Geometry check sheet. Reference: the model listing, model coordinates, mm. A direction names the side the tool comes from. Give positions to 0.01 mm unless a question says otherwise; leave off trailing zeros. Write each loop counter-clockwise with the first axis right and the second up, starting at its lowest first coordinate (ties: lowest second). Pieces come first, ordered by that corner, then holes. Notation, with made-up numbers: (20, -2.75) -> (67, -2.75) arc R28 ccw to (67, 32.25) -> close; hole circle Ø11 at (-39, 83.25). An arc over 180 degrees is marked (long way). Write item = value, one per line. Start each with the question number.
1. Thickness scan on line 1 along X through (y, z) = (89, -13.75); line 2 along X through (y, z) = (20.5, -13). Record the ranges inside material, lowest first.
2. Set-up check for faces 1 (the flat face through (-13, 62, -25)), 2 (the flat face through (-12, 65, -22)): record each of +Z, -Z, +X, -X, +Y, -Y from which the full face is reachable in a straight line by a thin tool's end or side.
3. Depth check by flat-ended pin: P1, Ø1.5, axis at x = -17, z = -2.5, coming from the -Y side. Enter the tip coordinate at first touch or a pass-through.
4. Mould release check, pull along X, two halves, no side actions. Record for faces 3 (the flat face through (-25, 74, -12)), 4 (the flat face through (0, 87, -13)), 5 (the flat face through (-22, 74, -13)): pulls with the +X half, pulls with the -X half, needs draft (parallel to the pull), parting line crosses it, or undercut.
5. Cross-section at B-B, the plane z = -7.25. Record the cut outline in (x, y).
6. Cross-section at A-A, the plane x = -9.75. Record the cut outline in (y, z), plus the area to 4 significant figures.
7. Cross-section at C-C, the plane y = 26.5. Record the cut outline in (x, z).
Autodesk Inventor part; units mm, degrees
ref_plane "YZ Plane" through (0, 0, 0) normal (1, 0, 0) x (0, 1, 0)
ref_plane "XZ Plane" through (0, 0, 0) normal (0, 1, 0) x (-1, 0, 0)
ref_plane "XY Plane" through (0, 0, 0) normal (0, 0, 1) x (1, 0, 0)
sketch "Sketch1" plane through (0, 0, 0) normal (0, 1, 0) x (-1, 0, 0)
  line L0 (0, 0) -> (25, 0)
  line L1 (25, 0) -> (25, -25)
  line L2 (25, -25) -> (0, -25)
  line L3 (0, -25) -> (0, 0)
  line L4 (22, -22) -> (22, -3)
  line L5 (22, -3) -> (3, -3)
  line L6 (3, -3) -> (3, -22)
  line L7 (3, -22) -> (22, -22)
  dimension "d0" = 25
  dimension "d1" = 25
  dimension "d2" = 3
extrude "Extrusion1" add sketch "Sketch1" along normal blind 150
sketch "Sketch2" plane through (0, 0, 0) normal (1, 0, 0) x (0, 0, -1)
  line L0 (0, 0) -> (25, 0)
  line L1 (25, 0) -> (25, 150)
  line L2 (0, 150) -> (25, 150)
  line L3 (0, 0) -> (0, 150)
  line L4 (0, 0) -> (0, 150)
  line L5 (0, 150) -> (25, 125)
  line L6 (0, 150) -> (35.3553, 150) construction
  dimension "d5" = 45
extrude "Extrusion2" cut sketch "Sketch2" against normal blind 80 contours L2 L1 L5
sketch "Sketch3" plane through (0, 0, -25) normal (0, 0, -1) x (-1, 0, 0)
  line L0 (25, 125) -> (0, 125)
  line L1 (0, 0) -> (0, 125)
  line L2 (0, 0) -> (25, 0)
  line L3 (25, 0) -> (25, 125)
  line L4 (25, 0) -> (0, 25)
  dimension "d11" = 45
extrude "Extrusion3" cut sketch "Sketch3" against normal blind 100 contours L2 L1 L4
properties part number "P405" material "Aluminum 6061"
Answers:
q1.line_1 = -25 to -22, -3 to 0
q1.line_2 = -25 to -22
q2.face_1 = -Z, +X, -X, +Y, -Y
q2.face_2 = +Y, -Y
q3.P1 = 7.25
q4.face_3 = pulls with the -X half
q4.face_4 = pulls with the +X half
q4.face_5 = undercut
q5.outline = (-25, 0) -> (-22, 3) -> (-22, 142.75) -> (-25, 142.75) -> close; (-3, 22) -> (0, 25) -> (0, 142.75) -> (-3, 142.75) -> close
q6.outline = (15.25, -25) -> (125, -25) -> (128, -22) -> (15.25, -22) -> close; (15.25, -3) -> (147, -3) -> (150, 0) -> (15.25, 0) -> close
q6.area = 733.5 mm^2
q7.outline = (-25, -25) -> (0, -25) -> (0, 0) -> (-25, 0) -> close; hole (-22, -22) -> (-3, -22) -> (-3, -3) -> (-22, -3) -> close
